Could you check a few things on this model? Use its own coordinates, in mm. A direction names the side the tool comes from. Give positions to 0.01 mm unless a question says otherwise; leave off trailing zeros. Write each loop counter-clockwise with the first axis right and the second up, starting at its lowest first coordinate (ties: lowest second). Pieces come first, ordered by that corner, then holes. Notation, with made-up numbers: (79.25, -8) -> (132.25, -8) arc R31 cw to (132.25, 30) -> close; hole circle Ø4 at (47, 20). An arc over 180 degrees is marked (long way). One line per question, with ' | ' between items.
from build123d import *

# Parameters (mm, degrees)
SKETCH1_W           = 70
SKETCH1_H           = 27
SKETCH1_R           = 0.5
BOSS_EXTRUDE2_DEPTH = 3
SKETCH2_W           = 70
SKETCH2_H           = 3
BOSS_EXTRUDE3_DEPTH = 25
SKETCH3_R           = 2.2
SKETCH3_W           = 42
SKETCH3_H           = 21
CUT_EXTRUDE1_DEPTH  = 25


with BuildPart() as part:
    # Sketch1 → Boss-Extrude2 (new body)
    with BuildSketch(Plane(origin=(0, 0, 0), x_dir=(1, 0, 0), z_dir=(0, 1, 0))):
        Rectangle(SKETCH1_W, SKETCH1_H)
        with Locations((-13.53, 0)):
            Circle(SKETCH1_R, mode=Mode.SUBTRACT)
        with Locations((0, 7.53)):
            Circle(SKETCH1_R, mode=Mode.SUBTRACT)
        with Locations((0, -7.53)):
            Circle(SKETCH1_R, mode=Mode.SUBTRACT)
        with Locations((13.53, 0)):
            Circle(SKETCH1_R, mode=Mode.SUBTRACT)
    extrude(amount=BOSS_EXTRUDE2_DEPTH)

    # Sketch2 → Boss-Extrude3 (add)
    with BuildSketch(Plane(origin=(0, 3, 0), x_dir=(1, 0, 0), z_dir=(0, 1, 0))):
        with Locations((0, -12)):
            Rectangle(SKETCH2_W, SKETCH2_H)
    extrude(amount=BOSS_EXTRUDE3_DEPTH)

    # Sketch3 → Cut-Extrude1 (cut)
    with BuildSketch(Plane.XY.offset(13.5)):
        with Locations((-24.89, 9)):
            Circle(SKETCH3_R)
        with Locations((-24.89, 19)):
            Circle(SKETCH3_R)
        with Locations((0, 14)):
            Rectangle(SKETCH3_W, SKETCH3_H)
        with Locations((24.89, 19)):
            Circle(SKETCH3_R)
        with Locations((24.89, 9)):
            Circle(SKETCH3_R)
    extrude(amount=-CUT_EXTRUDE1_DEPTH, mode=Mode.SUBTRACT)

    # Mirror1: part across plane


with BuildPart() as part_1:
    add(part.part)
    add(part.part.mirror(Plane.XY))


solid = part_1.part
Q1. Imagine slicing it at A-A on y = 9. Count the separate pieces of the cut face and the enclosed holes in it, and give its area (3 significant figures).
Answer below:
separate pieces: 8 | enclosed holes: 0 | area: 115 mm^2
Q2. Imagine slicing it at C-C on y = 23. Please give me the cut outline in (x, z).
Answer below:
outline: (-35, -13.5) -> (-21, -13.5) -> (-21, -10.5) -> (-35, -10.5) -> close; (-35, 10.5) -> (-21, 10.5) -> (-21, 13.5) -> (-35, 13.5) -> close; (21, -13.5) -> (35, -13.5) -> (35, -10.5) -> (21, -10.5) -> close; (21, 10.5) -> (35, 10.5) -> (35, 13.5) -> (21, 13.5) -> close
Q3. On a 3-axis mill with a long thin cutter (end or side, diameter ignored), from which of +Z, -Z, +X, -X, +Y, -Y can I reach the whole of each face in a straight line? I mean faces 1 (the flat face through (-21, 14, -12)), 2 (the flat face through (0, 26, 13.5)), 3 (the flat face through (0, 3, 0)). Say none if no direction works.
Answer below:
face 1: +Z, -Z | face 2: +Z, +X, -X, +Y, -Y | face 3: +X, -X, +Y
Q4. Imagine slicing it at B-B on x = 24.89. Please give me the cut outline in (y, z).
Answer below:
outline: (0, -13.5) -> (6.8, -13.5) -> (6.8, -10.5) -> (3, -10.5) -> (3, 10.5) -> (6.8, 10.5) -> (6.8, 13.5) -> (0, 13.5) -> close; (11.2, -13.5) -> (16.8, -13.5) -> (16.8, -10.5) -> (11.2, -10.5) -> close; (11.2, 10.5) -> (16.8, 10.5) -> (16.8, 13.5) -> (11.2, 13.5) -> close; (21.2, -13.5) -> (28, -13.5) -> (28, -10.5) -> (21.2, -10.5) -> close; (21.2, 10.5) -> (28, 10.5) -> (28, 13.5) -> (21.2, 13.5) -> close
Q5. If we mould it in two halves opening along X, with no side actions, what happens to faces 4 (the flat face through (0, 26, -13.5)), 5 (the flat face through (-35, 2.5, -1.1)), 6 (the cylindrical face through (-22.858, 8.157, 12.021))? For each: +X half, -X half, draft (parallel to the pull), parting line (faces both ways), or undercut.
Answer below:
face 4: draft | face 5: -X half | face 6: undercut
Q6. Imagine slicing it at D-D on x = -15. Please give me the cut outline in (y, z), and give its area (3 significant figures).
Answer below:
outline: (0, -13.5) -> (3.5, -13.5) -> (3.5, -10.5) -> (3, -10.5) -> (3, 10.5) -> (3.5, 10.5) -> (3.5, 13.5) -> (0, 13.5) -> close; (24.5, -13.5) -> (28, -13.5) -> (28, -10.5) -> (24.5, -10.5) -> close; (24.5, 10.5) -> (28, 10.5) -> (28, 13.5) -> (24.5, 13.5) -> close | area: 105 mm^2
Q7. If I drill on line 1 along Z through (x, y) = (0, 1.75); line 2 along Y through (x, z) = (24.89, 12.05); line 3 along X through (y, z) = (2.45, -7.53), over which ranges is the centre line in solid material (lowest first)?
Answer below:
line 1: z = -13.5 to -8.03, -7.03 to 7.03, 8.03 to 13.5 | line 2: y = 0 to 6.8, 11.2 to 16.8, 21.2 to 28 | line 3: x = -35 to -0.5, 0.5 to 35
